Autodesk Inventor part; units mm, degrees
ref_plane "YZ Plane" through (0, 0, 0) normal (1, 0, 0) x (0, 1, 0)
ref_plane "XZ Plane" through (0, 0, 0) normal (0, 1, 0) x (-1, 0, 0)
ref_plane "XY Plane" through (0, 0, 0) normal (0, 0, 1) x (1, 0, 0)
sketch "スケッチ1" plane through (0, 0, 0) normal (0, 1, 0) x (-1, 0, 0)
  line L0 (0, 0) -> (80, 0)
  line L1 (80, 0) -> (80, -142)
  line L2 (80, -142) -> (0, -142)
  line L3 (0, -142) -> (0, 0)
  dimension "d0" = 80
  dimension "d1" = 142
extrude "押し出し1" add sketch "スケッチ1" along normal blind 3.3
hole "穴1" at (-75.5, 3.3, -4.5) direction (0, -1, 0) diameter 3.4 end through all
hole "穴2" at (-4.5, 3.3, -4.5) direction (0, -1, 0) diameter 3.4 end through all
hole "穴3" at (-4.5, 3.3, -137.5) direction (0, -1, 0) diameter 3.4 end through all
hole "穴4" at (-75.5, 3.3, -137.5) direction (0, -1, 0) diameter 3.4 end through all
hole "穴5" at (-49, 3.3, -137.75) direction (0, -1, 0) diameter 2.4 end through all
hole "穴6" at (-31, 3.3, -137.75) direction (0, -1, 0) diameter 2.4 end through all
hole "穴7" at (-31, 3.3, -4.25) direction (0, -1, 0) diameter 2.4 end through all
hole "穴8" at (-49, 3.3, -4.25) direction (0, -1, 0) diameter 2.4 end through all
hole "穴9" at (-7, 0, -71) direction (0, 1, 0) diameter 2.4 end through all
hole "穴10" at (-23, 0, -71) direction (0, 1, 0) diameter 2.4 end through all
sketch "スケッチ3" plane through (0, 3.3, 0) normal (0, 1, 0) x (1, 0, 0)
  line L0 (0, 0) -> (0, 142)
  line L1 (0, 71) -> (-80, 71)
  line L2 (-80, 142) -> (-80, 0)
hole "穴15" at (-63.1, 3.3, -37) direction (0, -1, 0) diameter 2.4 end through all
ref_plane "作業平面1" through (0, 3.3, -71) normal (0, 0, -1) x (-1, 0, 0)
mirror "ミラー1" about plane through (0, 3.3, -71) normal (0, 0, -1) of "穴15"
properties part number "基本板(センサ1つ)" material "アルミニウム 5052"
Source: CAD feature listing. Evaluate the final solid. Frame: model axes, mm. Round coordinates to 2 decimals unless told otherwise and drop trailing zeros. Loops run counter-clockwise (first coordinate to the right, second up) from the corner with the lowest first, then second, coordinate; pieces in that order, holes last.
(1) Material intervals for probe 1 along Z at (x, y) = (-63.1, 2.2); probe 2 along Z at (x, y) = (-4.5, 1.75); probe 3 along X at (y, z) = (2.4, -4.25), sorted ascending.
From the geometry:
probe 1: z = -142 to -106.2, -103.8 to -38.2, -35.8 to 0
probe 2: z = -142 to -139.2, -135.8 to -6.2, -2.8 to 0
probe 3: x = -80 to -77.18, -73.82 to -50.2, -47.8 to -32.2, -29.8 to -6.18, -2.82 to 0
(2) Section query A-A (x = -75.5). Output: boundary loops of the cut face in (y, z).
From the geometry:
outline: (0, -142) - (3.3, -142) - (3.3, -139.2) - (0, -139.2) - close; (0, -135.8) - (3.3, -135.8) - (3.3, -6.2) - (0, -6.2) - close; (0, -2.8) - (3.3, -2.8) - (3.3, 0) - (0, 0) - close
(3) Contact query for flat-ended pins moving along their axis: pin 1 Ø2 at (x, z) = (-49, -4.25) entering from -Y; pin 2 Ø3 at (x, z) = (-63.1, -105) entering from +Y. Output: stop coordinate, or through.
From the geometry:
pin 1: passes through
pin 2: stops at y = 3.3
(4) Pull-direction query (X, two-part tool) for faces 1 (the flat face through (-39, 2, 0)), 2 (the flat face through (-80, 2, -70)), 3 (the flat face through (0, 2, -72)), 4 (the cylindrical face through (-76.01, 1.63, -135.88)); classes: +X half, -X half, draft (parallel to the pull), parting line (faces both ways), or undercut.
From the geometry:
face 1: draft
face 2: -X half
face 3: +X half
face 4: undercut
